```python
from build123d import *

# Parameters (mm, degrees)
SKETCH1_W           = 5
SKETCH1_H           = 30
SKETCH1_W_2         = 67.5
SKETCH1_H_2         = 5
BOSS_EXTRUDE1_DEPTH = 35
SKETCH2_R           = 1
CUT_EXTRUDE1_DEPTH  = 10
SKETCH3_W           = 60
SKETCH3_H           = 20
CUT_EXTRUDE2_DEPTH  = 10


with BuildPart() as part:
    # Sketch1 → Boss-Extrude1 (new, symmetric)
    with BuildSketch(Plane.XY):
        with Locations((-2.5, 15)):
            Rectangle(SKETCH1_W, SKETCH1_H)
        with Locations((33.75, 27.5)):
            Rectangle(SKETCH1_W_2, SKETCH1_H_2)
    extrude(amount=BOSS_EXTRUDE1_DEPTH, both=True)

    # Sketch2 → Cut-Extrude1 (cut)
    with BuildSketch(Plane.XZ):
        with Locations(Location((-2.5, 10, 0), (0, 0, 270))):
            Circle(SKETCH2_R)
        with Locations(Location((-2.5, -10, 0), (0, 0, 270))):
            Circle(SKETCH2_R)
    extrude(amount=-CUT_EXTRUDE1_DEPTH, mode=Mode.SUBTRACT)

    # Sketch3 → Cut-Extrude2 (cut)
    with BuildSketch(Plane.ZY.offset(5)):
        with Locations((0, 15)):
            Rectangle(SKETCH3_W, SKETCH3_H)
    extrude(amount=-CUT_EXTRUDE2_DEPTH, mode=Mode.SUBTRACT)


solid = part.part
```
Read the model definition and answer for the solid it produces. Units are mm, in the model's axes. A direction names the side the tool comes from. Give positions to 0.01 mm unless a question says otherwise; leave off trailing zeros. Write each loop counter-clockwise with the first axis right and the second up, starting at its lowest first coordinate (ties: lowest second). Pieces come first, ordered by that corner, then holes. Notation, with made-up numbers: (-29.5, 79) -> (20.5, 79) arc R21 ccw to (20.5, 107) -> close; hole circle Ø5 at (50.5, -1.5). An arc over 180 degrees is marked (long way). Answer as a JSON object with one key per item and string values.
1) Section C-C on z = 0 is taken. Write down the section's boundary in (x, y), then the cut area to 4 significant figures.
Findings below:
{"outline": "(-5, 0) -> (0, 0) -> (0, 5) -> (-5, 5) -> close; (-5, 25) -> (67.5, 25) -> (67.5, 30) -> (-5, 30) -> close", "area": "387.5 mm^2"}
2) Section A-A on z = 10 is taken. Write down the section's boundary in (x, y), then the cut area to 4 significant figures.
Findings below:
{"outline": "(-5, 0) -> (-3.5, 0) -> (-3.5, 5) -> (-5, 5) -> close; (-5, 25) -> (67.5, 25) -> (67.5, 30) -> (-5, 30) -> close; (-1.5, 0) -> (0, 0) -> (0, 5) -> (-1.5, 5) -> close", "area": "377.5 mm^2"}
3) A tool of negligible diameter and unlimited length cuts with its end or side. For faces 4 (the cylindrical face through (-3.1, 2.5, -9.2)), 5 (the flat face through (-3, 15, -30)), 6 (the flat face through (-5, 4.8, 0.5)), from which of +Z, -Z, +X, -X, +Y, -Y can it reach the whole face along a straight path? Write none if from no direction.
Findings below:
{"face 4": "-Y", "face 5": "+X, -X", "face 6": "+Z, -Z, -X, +Y, -Y"}
4) For a pull along Y with two mould halves and no side action, classify faces 1 (the flat face through (-3, 0, 0)), 2 (the flat face through (0, 4, 0)), 3 (the flat face through (-3, 15, 30)) as pulls with the +Y half, pulls with the -Y half, needs draft (parallel to the pull), parting line crosses it, or undercut.
Findings below:
{"face 1": "pulls with the -Y half", "face 2": "needs draft", "face 3": "undercut"}
5) Section B-B on y = 10.5 is taken. Write down the section's boundary in (x, z).
Findings below:
{"outline": "(-5, -35) -> (0, -35) -> (0, -30) -> (-5, -30) -> close; (-5, 30) -> (0, 30) -> (0, 35) -> (-5, 35) -> close"}
6) Section D-D on x = -2.5 is taken. Write down the section's boundary in (y, z), then the cut area to 3 significant figures.
Findings below:
{"outline": "(0, -35) -> (30, -35) -> (30, 35) -> (0, 35) -> (0, 11) -> (5, 11) -> (5, 30) -> (25, 30) -> (25, -30) -> (5, -30) -> (5, -11) -> (0, -11) -> close; (0, -9) -> (5, -9) -> (5, 9) -> (0, 9) -> close", "area": "880 mm^2"}
7) Flat-ended cylindrical pins translate along their axes: pin 1 Ø2 at (x, z) = (5, -27) entering from -Y; pin 2 Ø7.5 at (y, z) = (6.5, -5) entering from +X. Find the tip coordinate at first contact, or state that the pin passes through.
Findings below:
{"pin 1": "stops at y = 25", "pin 2": "stops at x = 0"}
8) Straight lines are drawn through the part: probe 1 along X at (y, z) = (1.65, 10); probe 2 along Y at (x, z) = (53, 28); probe 3 along X at (y, z) = (4, 26). For each, find the intervals that lie inside material, in ascending order. Write a range as from..to.
Findings below:
{"probe 1": "x = -5..-3.5, -1.5..0", "probe 2": "y = 25..30", "probe 3": "x = -5..0"}
